Geometry: final body of the model. Coordinates: model frame, mm. A direction names the side the tool comes from. Coordinates: 2 decimals unless noted, no trailing zeros. Loops run counter-clockwise (first coordinate to the right, second up) from the corner with the lowest first, then second, coordinate; pieces in that order, holes last. Notation, with made-up numbers: (73.5, 14) -> (105.5, 14) arc R4 cw to (105.5, 21) -> close; hole circle Ø9 at (3.5, -9.5). An arc over 180 degrees is marked (long way). One line per item, written item: value. Start each with the question number.
Item 1: Section query A-A on z = -10.16. Return loops of the section in (x, y) (1 decimal).
Item 2: Section query D-D on z = 32. Return loops of the section in (x, y) (3 decimals), then the cut area to 3 significant figures.
Item 3: Ray query, probe 1 along Z at (x, y) = (0, 5.25); probe 2 along X at (y, z) = (7.75, -10.16); probe 3 along Z at (x, y) = (-7, 6.5). Return the intervals inside material, ascending. Write a range as from..to.
Item 4: Mould query, pull axis X, two halves, no side actions, for faces 6 (the flat face through (5.759, 4.829, 79.184)), 7 (the flat face through (0, 9.525, 19)), 8 (the cylindrical face through (0.64, 4.696, 90.284)). Classes: +X half, -X half, draft (parallel to the pull), parting line (faces both ways), or undercut.
Item 5: Set-up query: faces 1 (the flat face through (-3.175, 5, 30)), 2 (the cylindrical face through (0.027, 4.829, 60.478)), 3 (the flat face through (7.938, 5, -26)), 4 (the flat face through (-7.938, 5, -25)), 5 (the flat face through (6, 5, 0)). Return all of +Z, -Z, +X, -X, +Y, -Y with unobstructed straight access to the full face (end or side cutting, diameter ignored); none if empty.
Item 6: Contact query for flat-ended pins moving along their axis: pin 1 Ø2 at (x, y) = (-9.5, 4) entering from +Z; pin 2 Ø5 at (y, z) = (4, 66) entering from -X; pin 3 Ø5 at (y, z) = (4.5, 19) entering from -X (3 decimals); pin 4 Ø5 at (x, z) = (3, -18) entering from -Y. Output: stop coordinate, or through.
Item 7: Section query C-C on y = 1.25. Give the number of separate pieces and of enclosed holes in the cut face, then the cut area to 3 significant figures.
Item 8: Section query B-B on x = 0. Return loops of the section in (y, z) (3 decimals).
from build123d import *

# Parameters (mm, degrees)
BOSS_EXTRUDE1_DEPTH = 9.525
SKETCH2_R           = 2.2479
CUT_EXTRUDE1_DEPTH  = 10.525
CUT_EXTRUDE2_DEPTH  = 10.525
FILLET1_R           = 1.25
FILLET2_R           = 2.54


with BuildPart() as part:
    # Sketch1 → Boss-Extrude1 (new body)
    with BuildSketch(Plane(origin=(0, 0, 0), x_dir=(1, 0, 0), z_dir=(0, 1, 0))):
        with BuildLine():
            Line((-7.9375, 50.8), (7.9375, 50.8))
            Line((7.9375, 50.8), (7.9375, 0))
            Line((7.9375, 0), (3.175, 0))
            Line((3.175, 0), (3.175, -58.867740133))
            ThreePointArc((3.175, -58.867740133), (0, -90.297), (-3.175, -58.867740133))
            Line((-3.175, -58.867740133), (-3.175, 0))
            Line((-3.175, 0), (-7.9375, 0))
            Line((-7.9375, 0), (-7.9375, 50.8))
        make_face()
    extrude(amount=BOSS_EXTRUDE1_DEPTH)

    # Sketch2 → Cut-Extrude1 (cut, through all)
    with BuildSketch(Plane(origin=(0, 9.525, 0), x_dir=(1, 0, 0), z_dir=(0, 1, 0))):
        with Locations((0, 40.64)):
            Circle(SKETCH2_R)
        with Locations((0, 10.16)):
            Circle(SKETCH2_R)
    extrude(amount=-CUT_EXTRUDE1_DEPTH, mode=Mode.SUBTRACT)

    # Sketch3 → Cut-Extrude2 (cut, through all)
    with BuildSketch(Plane(origin=(0, 9.525, 0), x_dir=(1, 0, 0), z_dir=(0, 1, 0))):
        with BuildLine():
            Line((0, -75.85914029), (10.376222628, -81.849855218))
            ThreePointArc((10.376222628, -81.849855218), (12.076377846, -81.3943), (11.620822628, -79.694144782))
            Line((11.620822628, -79.694144782), (1.2446, -73.703429855))
            Line((1.2446, -73.703429855), (1.2446, -61.722))
            ThreePointArc((1.2446, -61.722), (0, -60.4774), (-1.2446, -61.722))
            Line((-1.2446, -61.722), (-1.2446, -73.703429855))
            Line((-1.2446, -73.703429855), (-11.620822628, -79.694144782))
            ThreePointArc((-11.620822628, -79.694144782), (-12.076377846, -81.3943), (-10.376222628, -81.849855218))
            Line((-10.376222628, -81.849855218), (0, -75.85914029))
        make_face()
    extrude(amount=-CUT_EXTRUDE2_DEPTH, mode=Mode.SUBTRACT)

    # Fillet1
    fillet1_edges = [part.edges().sort_by_distance(p)[0] for p in [
        (-7.9375, 4.7625, -50.8),
        (7.9375, 4.7625, -50.8),
        (7.9375, 4.7625, 0),
        (3.175, 4.7625, 0),
        (3.175, 4.7625, 58.867740133),
        (-3.175, 4.7625, 58.867740133),
        (-3.175, 4.7625, 0),
        (-7.9375, 4.7625, 0),
    ]]
    fillet(fillet1_edges, radius=FILLET1_R)

    # Fillet2
    fillet2_edges = [part.edges().sort_by_distance(p)[0] for p in [
        (1.2446, 4.7625, 73.703429855),
        (0, 4.7625, 75.85914029),
        (-1.2446, 4.7625, 73.703429855),
    ]]
    fillet(fillet2_edges, radius=FILLET2_R)


solid = part.part
Reply:
1. outline: (-7.9, 0) -> (-2.2, 0) -> (-2.2, 9.5) -> (-7.9, 9.5) -> close; (2.2, 0) -> (7.9, 0) -> (7.9, 9.5) -> (2.2, 9.5) -> close
2. outline: (-3.175, 0) -> (3.175, 0) -> (3.175, 9.525) -> (-3.175, 9.525) -> close
2. area: 60.5 mm²
3. probe 1: z = -50.8..-42.89, -38.39..-12.41, -7.91..60.48, 76.25..90.3
3. probe 2: x = -7.94..-2.25, 2.25..7.94
3. probe 3: z = -50.76..-0.04, 60.17..77.03, 79.9..88.67
4. face 6: undercut
4. face 7: draft
4. face 8: parting line
5. face 1: -X, +Y, -Y
5. face 2: +Y, -Y
5. face 3: -Z, +X, +Y, -Y
5. face 4: -Z, -X, +Y, -Y
5. face 5: +X, +Y, -Y
6. pin 1: stops at z = 87.83
6. pin 2: stops at x = -14.73
6. pin 3: stops at x = -3.175
6. pin 4: stops at y = 0
7. separate pieces: 1
7. enclosed holes: 3
7. area: 1,840 mm²
8. outline: (0, -50.8) -> (9.525, -50.8) -> (9.525, -42.888) -> (0, -42.888) -> close; (0, -38.392) -> (9.525, -38.392) -> (9.525, -12.408) -> (0, -12.408) -> close; (0, -7.912) -> (9.525, -7.912) -> (9.525, 60.477) -> (0, 60.477) -> close; (0, 76.252) -> (9.525, 76.252) -> (9.525, 90.297) -> (0, 90.297) -> close
